from build123d import *

# Parameters (mm, degrees)
F0_W     = 132.1095339954
F0_H     = 70.0087491423
F1_DEPTH = 25.4
F2_W     = 132.1095339954
F2_H     = 11.6047412157
F3_DEPTH = 12.7
F4_W     = 132.1095339954
F4_H     = 11.0577493906
F5_DEPTH = 12.7
F6_W     = 62.4120058492
F6_H     = 47.346258536
F7_DEPTH = 20.32
F10_D    = 21.59
F12_D    = 21.59


with BuildPart() as f1:
    # F0 (on Top) → F1 (new body)
    with BuildSketch(Plane.XY):
        with Locations((-6.8613234907, -4.3028621003)):
            Rectangle(F0_W, F0_H)
    extrude(amount=F1_DEPTH)

    # F2 (on face) → F3 (cut)
    with BuildSketch(Plane.XY.offset(25.4)):
        with Locations((-6.8613234907, -33.5048660636)):
            Rectangle(F2_W, F2_H)
    extrude(amount=-F3_DEPTH, mode=Mode.SUBTRACT)

    # F4 (on face) → F5 (cut)
    with BuildSketch(Plane.XY.offset(25.4)):
        with Locations((-6.8613234907, 25.1726377755)):
            Rectangle(F4_W, F4_H)
    extrude(amount=-F5_DEPTH, mode=Mode.SUBTRACT)

    # F6 (on face) → F7 (join)
    with BuildSketch(Plane.XY.offset(25.4)):
        with Locations((-41.7100875638, -4.0293661878)):
            Rectangle(F6_W, F6_H)
    extrude(amount=F7_DEPTH)

    # F10 (through all)
    with Locations(Plane.XY.offset(45.72)):
        with Locations((-44.5797219872, -5.9616966173)):
            Hole(F10_D / 2)

    # F12 (through all)
    with Locations(Plane.XY.offset(25.4)):
        with Locations((22.5894171745, -6.0134478845)):
            Hole(F12_D / 2)


solid = f1.part
Build history of the part. All positions in model axes, mm. A direction names the side the tool comes from. Give positions to 0.01 mm unless a question says otherwise; leave off trailing zeros. Write each loop counter-clockwise with the first axis right and the second up, starting at its lowest first coordinate (ties: lowest second). Pieces come first, ordered by that corner, then holes. Notation, with made-up numbers: (-37.5, 31.25) - (7.5, 31.25) arc R10 ccw to (7.5, 35.25) - close; hole circle Ø2 at (37.5, 79). An arc over 180 degrees is marked (long way). Use one line per item in the form item = value. Start each with the question number.
1. Band-saw the part on D-D on z = 40.5. Write the cut outline in (x, y) (1 decimal), plus the area to 3 significant figures.
2. Drop flat-ended pins along their axis: pin 1 Ø12 at (x, y) = (20.5, 27.5) entering from +Z; pin 2 Ø6 at (x, y) = (45.5, 5.5) entering from +Z; pin 3 Ø10 at (x, z) = (11, 22) entering from -Y; pin 4 Ø1 at (x, y) = (45, -9) entering from -Z. Give the stop position or say it passes through.
3. Two-plate mould, pull along X, no slides. Class faces 1 (the face through (-8, -4, 0)), 2 (the face through (-10.504, -4, 35)), 3 (the face through (33.374, -5.539, 12.522)): released by +X, released by -X, zero draft, split by the parting line, or undercut.
4. Probe line 1 (X direction, y = -6.5, z = 43); line 2 (X direction, y = -1, z = 11); line 3 (X direction, y = -13, z = 7). List the from-to ranges inside material, lowest first. Write a range as [from, to].
5. Band-saw the part on A-A on y = 0. Write the cut outline in (x, z), plus the area to 3 significant figures.
6. Band-saw the part on B-B on x = -19. Write the cut outline in (y, z), plus the area to 3 significant figures.
7. 3-axis set-ups, long thin cutter, end or side, ignore diameter. For faces 4 (the face through (-8, -33, 12.7)), 5 (the face through (32, 2, 25.4)), 6 (the face through (-22, 19.644, 25)): which of +Z, -Z, +X, -X, +Y, -Y reach the whole face in a straight line?
8. Band-saw the part on C-C on x = -46. Write the cut outline in (y, z).
Conclusion:
q1.outline = (-72.9, -27.7) - (-10.5, -27.7) - (-10.5, 19.6) - (-72.9, 19.6) - close; hole circle Ø21.6 at (-44.6, -6)
q1.area = 2,590 mm²
q2.pin_1 = 12.7
q2.pin_2 = 25.4
q2.pin_3 = -27.7
q2.pin_4 = 0
q3.face_1 = zero draft
q3.face_2 = released by +X
q3.face_3 = undercut
q4.line_1 = [-72.92, -55.36], [-33.8, -10.5]
q4.line_2 = [-72.92, -54.17], [-34.99, 13.03], [32.15, 59.19]
q4.line_3 = [-72.92, -52.76], [-36.39, 14.36], [30.82, 59.19]
q5.outline = (-72.92, 0) - (-53.58, 0) - (-53.58, 45.72) - (-72.92, 45.72) - close; (-35.58, 0) - (13.62, 0) - (13.62, 25.4) - (-10.5, 25.4) - (-10.5, 45.72) - (-35.58, 45.72) - close; (31.55, 0) - (59.19, 0) - (59.19, 25.4) - (31.55, 25.4) - close
q5.area = 3,350 mm²
q6.outline = (-39.31, 0) - (30.7, 0) - (30.7, 12.7) - (19.64, 12.7) - (19.64, 45.72) - (-27.7, 45.72) - (-27.7, 12.7) - (-39.31, 12.7) - close
q6.area = 2,450 mm²
q7.face_4 = +Z, +X, -X, -Y
q7.face_5 = +Z, +X, +Y, -Y
q7.face_6 = +Z, +X, -X, +Y
q8.outline = (-39.31, 0) - (-16.66, 0) - (-16.66, 45.72) - (-27.7, 45.72) - (-27.7, 12.7) - (-39.31, 12.7) - close; (4.74, 0) - (30.7, 0) - (30.7, 12.7) - (19.64, 12.7) - (19.64, 45.72) - (4.74, 45.72) - close
